Check sheet for the modelled part. Datum: model origin and axes. Units: mm. Face numbers are marked on the shaded views. Round coordinates to 2 decimals unless told otherwise and drop trailing zeros.
(1) Mould release check, pull along Y, two halves, no side actions. Record for the marked faces 1 and 2: released by +Y, released by -Y, zero draft, split by the parting line, or undercut.
(2) Depth check by flat-ended pin: pin 1 (5 mm diameter, centred on y = -79.375, z = -13.2, fed in from +X); pin 2 (2 mm diameter, centred on x = 2.5, z = -60.5, fed in from -Y); pin 3 (6 mm diameter, centred on y = 91, z = -3.5, fed in from -X); pin 4 (2 mm diameter, centred on x = 13.5, y = 7, fed in from +Z). Enter the tip coordinate at first touch or a pass-through.
(3) Thickness scan on probe 1 along Y at (x, z) = (0.5, -4.5); probe 2 along Y at (x, z) = (6, -31); probe 3 along X at (y, z) = (-62, -96). Record the ranges inside material, lowest first.
(4) Sectioned sample at A-A, the plane z = -38.6. Count the separate pieces of the cut face and the enclosed holes in it, and give its area (3 significant figures).
```python
from build123d import *

# Parameters (mm, degrees)
REVOLVE_THIN1_ANGLE               = 180
SKETCH81_W                        = 41.373480097
SKETCH81_H                        = 433.466768404
EXTRUDE1_DEPTH                    = 22.75344145
EXTRUDE1_DEPTH_BACK               = 4.64655855
BOSS_EXTRUDE1_DEPTH               = 25.4
CUT_EXTRUDE1_DEPTH                = 6.35
F_5_16_CLEARANCE_HOLE1_AT_2_COUNT = 2
F_5_16_CLEARANCE_HOLE1_AT_2_PITCH = 25.4
F_5_16_CLEARANCE_HOLE1_AT_3_COUNT = 2
F_5_16_CLEARANCE_HOLE1_AT_3_PITCH = 158.75
F_5_16_CLEARANCE_HOLE1_AT_4_COUNT = 2
F_5_16_CLEARANCE_HOLE1_AT_4_PITCH = 161.247301583
CUT_EXTRUDE2_DEPTH                = 8.25
CUT_EXTRUDE3_DEPTH                = 2.5034
FILLET1_R                         = 4.7625
FILLET2_R                         = 4.7625
SKETCH88_W                        = 10
SKETCH88_H                        = 6.35254
CUT_EXTRUDE4_DEPTH                = 6.35
SKETCH89_W                        = 10
SKETCH89_H                        = 7.35254
CUT_EXTRUDE5_DEPTH                = 6.35
FILLET3_R                         = 3.175


with BuildPart() as part:
    # Sketch1 → Revolve-Thin1 (revolve)
    with BuildSketch(Plane.XY):
        with BuildLine():
            Line((21.75344145, 119.175), (13.030353167, 119.175))
            ThreePointArc((13.030353167, 119.175), (10.546995544, 116.615384298), (7.1068829, 115.675))
            Line((7.1068829, 115.675), (-3.64655855, 115.675))
            Line((-3.64655855, 115.675), (-3.64655855, 109.325))
            Line((-3.64655855, 109.325), (7.1068829, 109.325))
            ThreePointArc((7.1068829, 109.325), (11.897172557, 110.231322005), (16.025262798, 112.825))
            Line((16.025262798, 112.825), (21.75344145, 112.825))
            Line((21.75344145, 112.825), (21.75344145, 119.175))
        make_face()
    revolve(axis=Axis((0, 0, 0), (-1, 0, 0)), revolution_arc=REVOLVE_THIN1_ANGLE)

    # Sketch81 → Extrude1 (cut, two sides)
    with BuildSketch(Plane(origin=(0, 0, 0), x_dir=(0, 0, -1), z_dir=(1, 0, 0))) as extrude1_sk:
        with Locations((-20.186740049, 1.572115024)):
            Rectangle(SKETCH81_W, SKETCH81_H)
    extrude(amount=EXTRUDE1_DEPTH, mode=Mode.SUBTRACT)
    extrude(extrude1_sk.sketch, amount=-EXTRUDE1_DEPTH_BACK, mode=Mode.SUBTRACT)

    # Sketch82 → Boss-Extrude1 (add)
    with BuildSketch(Plane(origin=(21.75344145, 0, 0), x_dir=(0, 0, -1), z_dir=(1, 0, 0))):
        with BuildLine():
            Line((0.5, 112.823892084), (0.5, 68.373171822))
            ThreePointArc((0.5, 68.373171822), (68.375, 0), (0.5, -68.373171822))
            Line((0.5, -68.373171822), (0.5, -112.823892084))
            ThreePointArc((0.5, -112.823892084), (112.825, 0), (0.5, 112.823892084))
        make_face()
    extrude(amount=-BOSS_EXTRUDE1_DEPTH)

    # Sketch83 → Cut-Extrude1 (cut)
    with BuildSketch(Plane(origin=(21.75344145, 0, 0), x_dir=(0, 0, -1), z_dir=(1, 0, 0))):
        with BuildLine():
            Line((0.5, -68.373171822), (0.5, -119.173951118))
            ThreePointArc((0.5, -119.173951118), (119.175, 0), (0.5, 119.173951118))
            Line((0.5, 119.173951118), (0.5, 68.373171822))
            ThreePointArc((0.5, 68.373171822), (68.375, 0), (0.5, -68.373171822))
        make_face()
    extrude(amount=-CUT_EXTRUDE1_DEPTH, mode=Mode.SUBTRACT)

    # Sketch84 → 5_16 Clearance Hole1 (revolve, cut)
    with BuildSketch(Plane(origin=(-3.64655855, -79.375, -38.6), x_dir=(0, 0, 1), z_dir=(0, 1, 0))):
        Polygon((0, 0), (0, 19.05), (4.7371, 19.05), (4.1021, 18.415), (4.1021, 0.635), (4.7371, 0), align=None)
    f_5_16_clearance_hole1 = revolve(axis=Axis((-9.99655855, -79.375, -38.6), (1, 0, 0)), mode=Mode.SUBTRACT)

    # 5_16 Clearance Hole1 at 2: 5_16 Clearance Hole1 ×2
    with Locations(*[(0, 0, i * F_5_16_CLEARANCE_HOLE1_AT_2_PITCH) for i in range(1, F_5_16_CLEARANCE_HOLE1_AT_2_COUNT)]):
        add(f_5_16_clearance_hole1, mode=Mode.SUBTRACT)

    # 5_16 Clearance Hole1 at 3: 5_16 Clearance Hole1 ×2
    with Locations(*[(0, i * F_5_16_CLEARANCE_HOLE1_AT_3_PITCH, 0) for i in range(1, F_5_16_CLEARANCE_HOLE1_AT_3_COUNT)]):
        add(f_5_16_clearance_hole1, mode=Mode.SUBTRACT)

    # 5_16 Clearance Hole1 at 4: 5_16 Clearance Hole1 ×2
    with Locations(*[Vector(0, 0.984512599, 0.175313838) * (i * F_5_16_CLEARANCE_HOLE1_AT_4_PITCH) for i in range(1, F_5_16_CLEARANCE_HOLE1_AT_4_COUNT)]):
        add(f_5_16_clearance_hole1, mode=Mode.SUBTRACT)

    # Sketch86 → Cut-Extrude2 (cut)
    with BuildSketch(Plane.ZY.offset(3.64655855)):
        with BuildLine():
            Line((-22.551231845, 113.455487163), (-20.694300932, 104.113247999))
            ThreePointArc((-20.694300932, 104.113247999), (-13.855355304, 105.241872035), (-6.957331702, 105.921754308))
            Line((-6.957331702, 105.921754308), (-7.581623596, 115.426273476))
            ThreePointArc((-7.581623596, 115.426273476), (-15.098617285, 114.685384339), (-22.551231845, 113.455487163))
        make_face()
        with BuildLine():
            Line((-22.893664129, 103.651833765), (-24.947947227, 112.952669531))
            ThreePointArc((-24.947947227, 112.952669531), (-81.791721695, 81.797432033), (-112.95092756, 24.95583275))
            Line((-112.95092756, 24.95583275), (-103.650235233, 22.900900336))
            ThreePointArc((-103.650235233, 22.900900336), (-75.05676471, 75.062004844), (-22.893664129, 103.651833765))
        make_face()
        with BuildLine():
            Line((-113.455487163, 22.551231845), (-104.113247999, 20.694300932))
            ThreePointArc((-104.113247999, 20.694300932), (-105.241872035, 13.855355304), (-105.921754308, 6.957331702))
            Line((-105.921754308, 6.957331702), (-115.426273476, 7.581623596))
            ThreePointArc((-115.426273476, 7.581623596), (-114.685384339, 15.098617285), (-113.455487163, 22.551231845))
        make_face()
        with BuildLine():
            Line((-115.561262836, 5.128367845), (-106.045628269, 4.706083827))
            ThreePointArc((-106.045628269, 4.706083827), (-84.214457072, -64.620025689), (-22.900900336, -103.650235233))
            Line((-22.900900336, -103.650235233), (-24.95583275, -112.95092756))
            ThreePointArc((-24.95583275, -112.95092756), (-91.771147638, -70.418478301), (-115.561262836, 5.128367845))
        make_face()
        with BuildLine():
            Line((-22.551231845, -113.455487163), (-20.694300932, -104.113247999))
            ThreePointArc((-20.694300932, -104.113247999), (-13.855355304, -105.241872035), (-6.957331702, -105.921754308))
            Line((-6.957331702, -105.921754308), (-7.581623596, -115.426273476))
            ThreePointArc((-7.581623596, -115.426273476), (-15.098617285, -114.685384339), (-22.551231845, -113.455487163))
        make_face()
    extrude(amount=-CUT_EXTRUDE2_DEPTH, mode=Mode.SUBTRACT)

    # Sketch87 → Cut-Extrude3 (cut)
    with BuildSketch(Plane.ZY.offset(-4.60344145)):
        with BuildLine():
            Line((-24.95583275, -112.95092756), (-22.900900336, -103.650235233))
            ThreePointArc((-22.900900336, -103.650235233), (-84.214457072, -64.620025689), (-106.045628269, 4.706083827))
            Line((-106.045628269, 4.706083827), (-115.561262836, 5.128367845))
            ThreePointArc((-115.561262836, 5.128367845), (-91.771147638, -70.418478301), (-24.95583275, -112.95092756))
        make_face()
        with BuildLine():
            Line((-22.893664129, 103.651833765), (-24.947947227, 112.952669531))
            ThreePointArc((-24.947947227, 112.952669531), (-81.791721695, 81.797432033), (-112.95092756, 24.95583275))
            Line((-112.95092756, 24.95583275), (-103.650235233, 22.900900336))
            ThreePointArc((-103.650235233, 22.900900336), (-75.05676471, 75.062004844), (-22.893664129, 103.651833765))
        make_face()
    extrude(amount=-CUT_EXTRUDE3_DEPTH, mode=Mode.SUBTRACT)

    # Fillet1
    fillet1_edges = [part.edges().sort_by_distance(p)[0] for p in [
        (0.47844145, 105.921754308, -6.957331702),
        (0.47844145, 104.113247999, -20.694300932),
        (1.73014145, 103.651833765, -22.893664129),
        (1.73014145, 22.900900336, -103.650235233),
        (0.47844145, 20.694300932, -104.113247999),
        (0.47844145, 6.957331702, -105.921754308),
        (1.73014145, 4.706083827, -106.045628269),
        (1.73014145, -103.650235233, -22.900900336),
        (0.47844145, -104.113247999, -20.694300932),
        (0.47844145, -105.921754308, -6.957331702),
    ]]
    fillet(fillet1_edges, radius=FILLET1_R)

    # Fillet2
    fillet2_edges = [part.edges().sort_by_distance(p)[0] for p in [
        (7.10684145, -110.575810848, -24.4310649),
        (7.10684145, 24.4310649, -110.575810848),
        (7.10684145, 110.577516189, -24.423345192),
        (7.10684145, 75.062004844, -75.05676471),
        (7.10684145, 24.487736641, -104.698272262),
        (7.10684145, 104.699981573, -24.480427263),
        (7.10684145, 5.020529225, -113.131256349),
        (7.10684145, -64.620025689, -84.214457072),
        (7.10684145, -104.698272262, -24.487736641),
        (7.10684145, 3.444569602, -107.468657759),
    ]]
    fillet(fillet2_edges, radius=FILLET2_R)

    # Sketch88 → Cut-Extrude4 (cut)
    with BuildSketch(Plane.ZY.offset(3.64655855)):
        with Locations((-5.5, -90)):
            Rectangle(SKETCH88_W, SKETCH88_H)
        with Locations((-5.5, 90)):
            Rectangle(SKETCH88_W, SKETCH88_H)
    extrude(amount=-CUT_EXTRUDE4_DEPTH, mode=Mode.SUBTRACT)

    # Sketch89 → Cut-Extrude5 (cut)
    with BuildSketch(Plane.ZY.offset(3.64655855)):
        with Locations((-5.5, 90)):
            Rectangle(SKETCH89_W, SKETCH89_H)
    extrude(amount=-CUT_EXTRUDE5_DEPTH, mode=Mode.SUBTRACT)

    # Fillet3
    fillet3_edges = [part.edges().sort_by_distance(p)[0] for p in [
        (-0.47155855, -93.17627, -10.5),
        (-0.47155855, -86.82373, -10.5),
        (-0.47155855, 86.32373, -10.5),
        (-0.47155855, 93.67627, -10.5),
    ]]
    fillet(fillet3_edges, radius=FILLET3_R)


solid = part.part
```
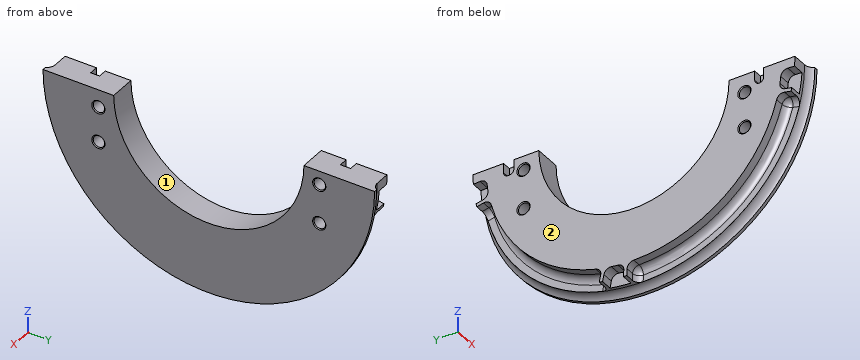
Derived:
1. face 1: undercut
1. face 2: zero draft
2. pin 1: passes through
2. pin 2: stops at y = -87.91
2. pin 3: stops at x = -3.65
2. pin 4: stops at z = -67.91
3. probe 1: y = -115.59 to -93.18, -86.82 to -68.23, 68.23 to 86.32, 93.68 to 115.59
3. probe 2: y = -103.31 to -60.94, 60.94 to 103.31
3. probe 3: x = 7.11 to 15.4
4. separate pieces: 4
4. enclosed holes: 0
4. area: 1,510 mm2
